from build123d import *

# Parameters (mm, degrees)
EXTRUDE_1_DEPTH     = 8
FILLET_1_R          = 8
CUT_EXTRUDE_1_DEPTH = 1
SKETCH_3_R          = 2.5
EXTRUDE_2_DEPTH     = 4
SKETCH_4_R          = 4
CUT_EXTRUDE_3_DEPTH = 1
CUT_EXTRUDE_4_REACH = 13
SKETCH_5_R          = 2.5
CUT_EXTRUDE_START   = -7
SKETCH_4_2_R        = 4
CUT_EXTRUDE_5_DEPTH = 2
SKETCH_7_R          = 4
CUT_EXTRUDE_6_DEPTH = 1
FILLET_2_R          = 2
SKETCH_9_R          = 5
EXTRUDE_3_DEPTH     = 8
SKETCH_11_R         = 3
EXTRUDE_4_DEPTH     = 2.5
FILLET_3_R          = 1
SKETCH_12_R         = 1.6
CUT_EXTRUDE_8_DEPTH = 12
CUT_EXTRUDE_9_DEPTH = 4


with BuildPart() as part:
    # 草图1 → 凸台-拉伸1 (new body)
    with BuildSketch(Plane.XY):
        with BuildLine():
            Line((-5, -175), (-5, -180))
            ThreePointArc((-5, -180), (0, -185), (5, -180))
            Line((5, -180), (5, -175))
            Line((5, -175), (10, -170))
            Line((10, -170), (10, -140))
            Line((10, -140), (5, -135))
            Line((5, -135), (5, 0))
            ThreePointArc((5, 0), (0, 5), (-5, 0))
            Line((-5, 0), (-5, -135))
            Line((-5, -135), (0, -140))
            Line((0, -140), (0, -170))
            Line((0, -170), (-5, -175))
        make_face()
    extrude(amount=EXTRUDE_1_DEPTH)

    # 圆角1
    fillet_1_edges = [part.edges().sort_by_distance(p)[0] for p in [
        (5, -175, 4),
        (-5, -175, 4),
        (0, -170, 4),
        (0, -140, 4),
        (-5, -135, 4),
        (5, -135, 4),
        (10, -140, 4),
        (10, -170, 4),
    ]]
    fillet(fillet_1_edges, radius=FILLET_1_R)

    # 草图2 → 切除-拉伸1 (cut)
    with BuildSketch(Plane(origin=(0, 0, 0), x_dir=(-1, 0, 0), z_dir=(0, 0, -1))):
        with BuildLine():
            Line((5, 0), (5, -2.75))
            Line((5, -2.75), (4.763139721, -2.75))
            ThreePointArc((4.763139721, -2.75), (0, -5.5), (-4.763139721, -2.75))
            Line((-4.763139721, -2.75), (-5, -2.75))
            Line((-5, -2.75), (-5, 0))
            ThreePointArc((-5, 0), (0, 5), (5, 0))
        make_face()
    extrude(amount=-CUT_EXTRUDE_1_DEPTH, mode=Mode.SUBTRACT)

    # 草图3 → 凸台-拉伸2 (add)
    with BuildSketch(Plane(origin=(0, 0, 1), x_dir=(-1, 0, 0), z_dir=(0, 0, -1))):
        Circle(SKETCH_3_R)
    extrude(amount=EXTRUDE_2_DEPTH)

    # 草图4 → 切除-拉伸3 (cut)
    with BuildSketch(Plane(origin=(0, 0, 1), x_dir=(-1, 0, 0), z_dir=(0, 0, -1))):
        with BuildLine():
            Line((-5, 0), (-5, -2.75))
            Line((-5, -2.75), (-4.763139721, -2.75))
            ThreePointArc((-4.763139721, -2.75), (0, -5.5), (4.763139721, -2.75))
            Line((4.763139721, -2.75), (5, -2.75))
            Line((5, -2.75), (5, 0))
            ThreePointArc((5, 0), (0, 5), (-5, 0))
        make_face()
        Circle(SKETCH_4_R, mode=Mode.SUBTRACT)
    extrude(amount=-CUT_EXTRUDE_3_DEPTH, mode=Mode.SUBTRACT)

    # 草图5 → 切除-拉伸4 (cut, up to next)
    with BuildSketch(Plane.XY.offset(8), mode=Mode.PRIVATE) as cut_extrude_4_sk1:
        Circle(SKETCH_5_R)
    cut_extrude_4_tool1 = extrude(cut_extrude_4_sk1.sketch, amount=-CUT_EXTRUDE_4_REACH, mode=Mode.PRIVATE) & part.part
    add(cut_extrude_4_tool1.solids().sort_by_distance((0, 0, 8))[0], mode=Mode.SUBTRACT)

    # 草图4<2> → 切除-拉伸5 (cut)
    with BuildSketch(Plane(origin=(0, 0, 1), x_dir=(-1, 0, 0), z_dir=(0, 0, -1)).offset(CUT_EXTRUDE_START)):
        with BuildLine():
            Line((-5, 0), (-5, -2.75))
            Line((-5, -2.75), (-4.763139721, -2.75))
            ThreePointArc((-4.763139721, -2.75), (0, -5.5), (4.763139721, -2.75))
            Line((4.763139721, -2.75), (5, -2.75))
            Line((5, -2.75), (5, 0))
            ThreePointArc((5, 0), (0, 5), (-5, 0))
        make_face()
        Circle(SKETCH_4_2_R, mode=Mode.SUBTRACT)
    extrude(amount=CUT_EXTRUDE_5_DEPTH, mode=Mode.SUBTRACT)

    # 草图7 → 切除-拉伸6 (cut)
    with BuildSketch(Plane.XY.offset(8)):
        Circle(SKETCH_7_R)
    extrude(amount=-CUT_EXTRUDE_6_DEPTH, mode=Mode.SUBTRACT)

    # 圆角2
    fillet_2_edges = [part.edges().sort_by_distance(p)[0] for p in [
        (-4.39103626, -134.74775896, 0),
        (-2.5, -137.5, 0),
        (-0.60896374, -140.25224104, 0),
        (0, -155, 0),
        (-0.60896374, -169.74775896, 0),
        (-2.5, -172.5, 0),
        (-4.39103626, -175.25224104, 0),
        (-5, -179.156854249, 0),
        (0, -185, 0),
        (5, -179.156854249, 0),
        (5.60896374, -175.25224104, 0),
        (7.5, -172.5, 0),
        (9.39103626, -169.74775896, 0),
        (10, -155, 0),
        (9.39103626, -140.25224104, 0),
        (7.5, -137.5, 0),
        (5.60896374, -134.74775896, 0),
        (-4.39103626, -134.74775896, 8),
        (-2.5, -137.5, 8),
        (-0.60896374, -140.25224104, 8),
        (0, -155, 8),
        (-0.60896374, -169.74775896, 8),
        (-2.5, -172.5, 8),
        (-4.39103626, -175.25224104, 8),
        (-5, -179.156854249, 8),
        (0, -185, 8),
        (5, -179.156854249, 8),
        (5.60896374, -175.25224104, 8),
        (7.5, -172.5, 8),
        (9.39103626, -169.74775896, 8),
        (10, -155, 8),
        (9.39103626, -140.25224104, 8),
        (7.5, -137.5, 8),
        (5.60896374, -134.74775896, 8),
        (-5, -67.218145751, 0),
        (5, -67.218145751, 0),
        (-5, -67.218145751, 8),
        (5, -67.218145751, 8),
    ]]
    fillet(fillet_2_edges, radius=FILLET_2_R)

    # 草图9 → 凸台-拉伸3 (add)
    with BuildSketch(Plane.XY.offset(8)):
        with Locations((0, -180)):
            Circle(SKETCH_9_R)
    extrude(amount=-EXTRUDE_3_DEPTH)

    # 草图11 → 凸台-拉伸4 (add)
    with BuildSketch(Plane(origin=(0, 0, 0), x_dir=(-1, 0, 0), z_dir=(0, 0, -1))):
        with Locations((0, -180)):
            Circle(SKETCH_11_R)
    extrude(amount=EXTRUDE_4_DEPTH)

    # 圆角3
    fillet_3_edges = [part.edges().sort_by_distance(p)[0] for p in [
        (3, -180, 0),
    ]]
    fillet(fillet_3_edges, radius=FILLET_3_R)

    # 草图12 → 切除-拉伸8 (cut)
    with BuildSketch(Plane(origin=(0, 0, -2.5), x_dir=(-1, 0, 0), z_dir=(0, 0, -1))):
        with Locations((0, -180)):
            Circle(SKETCH_12_R)
    extrude(amount=-CUT_EXTRUDE_8_DEPTH, mode=Mode.SUBTRACT)

    # 草图13 → 切除-拉伸9 (cut)
    with BuildSketch(Plane.XY.offset(8)):
        Polygon((-1.58771324, -177.25), (-3.175426481, -180), (-1.58771324, -182.75), (1.58771324, -182.75), (3.175426481, -180), (1.58771324, -177.25), align=None)
    extrude(amount=-CUT_EXTRUDE_9_DEPTH, mode=Mode.SUBTRACT)


solid = part.part
Can you work these out from the model? Positions are in its coordinate system, mm. A direction names the side the tool comes from. Give positions to 0.01 mm unless a question says otherwise; leave off trailing zeros. Loops run counter-clockwise (first coordinate to the right, second up) from the corner with the lowest first, then second, coordinate; pieces in that order, holes last. Notation, with made-up numbers: (62.25, 16.5) - (96.25, 16.5) arc R22 cw to (96.25, 48.5) - close; hole circle Ø3 at (35, 12). An arc over 180 degrees is marked (long way). One line per item, written item: value.
(1) If we section it at A-A, the plane y = -44.5: List the corners of the cut face in (x, z) for me, plus the area to 3 significant figures.
Verdict:
outline: (-5, 2) arc R2 ccw to (-3, 0) - (3, 0) arc R2 ccw to (5, 2) - (5, 6) arc R2 ccw to (3, 8) - (-3, 8) arc R2 ccw to (-5, 6) - close
area: 76.6 mm^2
(2) I need wall thicknesses on line 1 along X through (y, z) = (-180, 2); line 2 along Z through (x, y) = (2.75, -62); line 3 along X through (y, z) = (-105, 5.5). Which ranges of each line are inside material? Lowest first, please.
Verdict:
line 1: -5 to -1.6, 1.6 to 5
line 2: 0 to 8
line 3: -5 to 5
(3) On a 3-axis mill with a long thin cutter (end or side, diameter ignored), from which of +Z, -Z, +X, -X, +Y, -Y can I reach the whole of each face in a straight line? I mean faces 1 (the face through (0, -155, 4)), 2 (the face through (0, -177, -2)), 3 (the face through (0, -182.75, 6)). Say none if no direction works.
Verdict:
face 1: +Z, -Z, -X
face 2: -Z
face 3: +Z
(4) If we mould it in two halves opening along X, with no side actions, what happens to faces 4 (the face through (-0.592, -169.707, 4.028)), 5 (the face through (0.867, -3.905, 6.507)), 6 (the face through (0.867, -3.905, 1.493)), 7 (the face through (5.592, -175.293, 4.028))? For each: released by +X, released by -X, zero draft, split by the parting line, or undercut.
Verdict:
face 4: released by -X
face 5: undercut
face 6: undercut
face 7: released by +X
(5) I'm going to push flat-ended pins straight in: pin 1 (8 mm diameter, centred on x = 0, y = 0, fed in from +Z); pin 2 (4.5 mm diameter, centred on y = -79, z = 3, fed in from +X); pin 3 (4 mm diameter, centred on x = -3, z = 6.5, fed in from +Y). Where does each tip first touch, or does it pass through?
Verdict:
pin 1: z = 7
pin 2: x = 5
pin 3: y = 4.89
